Verification items for this drawing (mm, ordinates from the low corner). A direction names the side the tool comes from. Coordinates: 2 decimals unless noted, no trailing zeros. Order: outer loops, then holes, each group sorted by start corner. A loop starts at its lowest first (then second) coordinate and runs counter-clockwise, first axis right, second up. Notation, with made-up numbers: M -22.75,30.25 L 4.25,30.25 A21 cw 4.25,35.25 Z; hole C -32,-3.75 d5. An arc over 180 degrees is marked long. Write item = value, one per line.
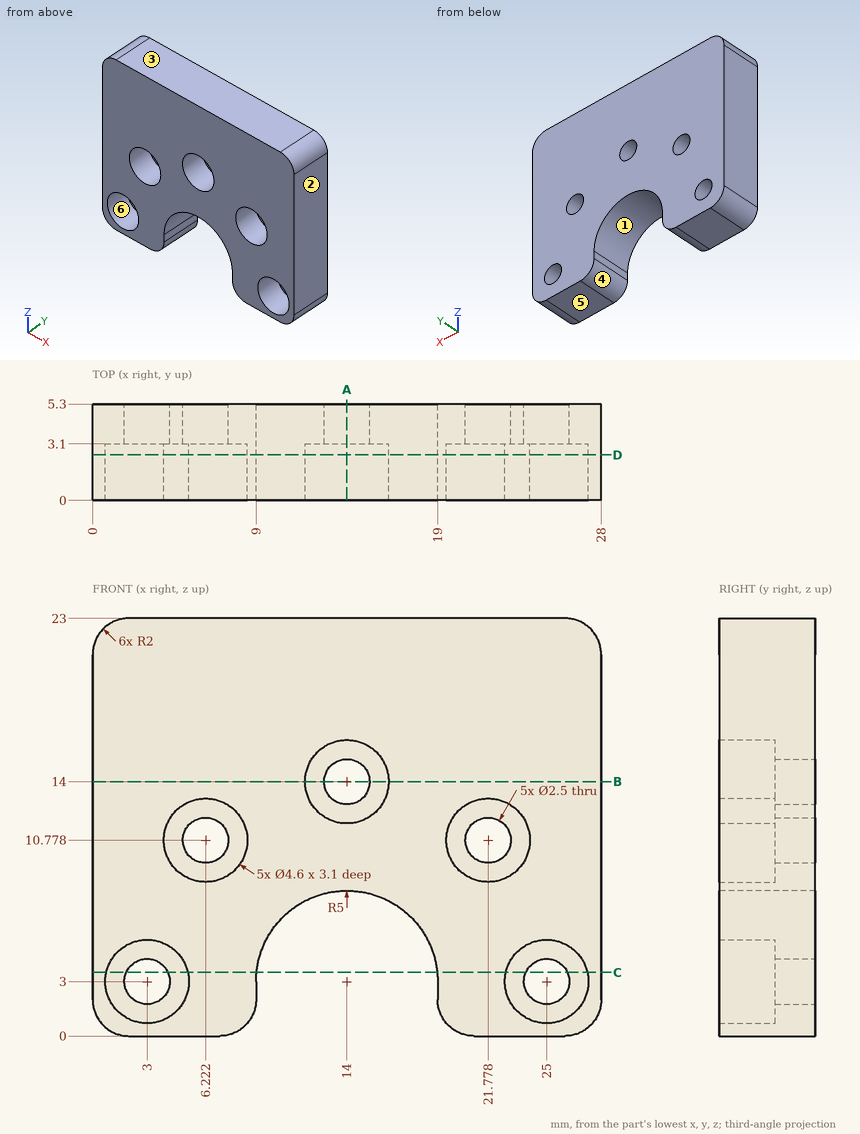
Item 1: Tool access check on the marked faces 4, 5 and 6. Record the directions out of +Z, -Z, +X, -X, +Y, -Y that give a thin tool (end or side, any length) a straight path to the whole face; none if there is none.
Report:
face_4 = -Z, +Y, -Y
face_5 = -Z, +X, -X, +Y, -Y
face_6 = -Y
Item 2: Release check for a two-part mould opening along X. For the marked faces 1, 2 and 3 record: pulls with the +X half, pulls with the -X half, needs draft (parallel to the pull), parting line crosses it, or undercut.
Report:
face_1 = undercut
face_2 = pulls with the +X half
face_3 = needs draft
Item 3: Sectioned sample at A-A, the plane x = 14. Enter the section's corners in (y, z).
Report:
outline = M 0,8 L 5.3,8 L 5.3,12.75 L 3.1,12.75 L 3.1,11.7 L 0,11.7 Z; M 0,16.3 L 3.1,16.3 L 3.1,15.25 L 5.3,15.25 L 5.3,23 L 0,23 Z
Item 4: Sectioned sample at C-C, the plane z = 3.5. Enter the section's corners in (x, y) (1 decimal).
Report:
outline = M 0,0 L 0.8,0 L 0.8,3.1 L 1.9,3.1 L 1.9,5.3 L 0,5.3 Z; M 4.1,3.1 L 5.2,3.1 L 5.2,0 L 9,0 L 9,5.3 L 4.1,5.3 Z; M 19,0 L 22.8,0 L 22.8,3.1 L 23.9,3.1 L 23.9,5.3 L 19,5.3 Z; M 26.1,3.1 L 27.2,3.1 L 27.2,0 L 28,0 L 28,5.3 L 26.1,5.3 Z
Item 5: Sectioned sample at B-B, the plane z = 14. Enter the section's corners in (x, y).
Report:
outline = M 0,0 L 11.7,0 L 11.7,3.1 L 12.75,3.1 L 12.75,5.3 L 0,5.3 Z; M 15.25,3.1 L 16.3,3.1 L 16.3,0 L 28,0 L 28,5.3 L 15.25,5.3 Z
Item 6: Sectioned sample at D-D, the plane y = 2.5. Enter the section's corners in (x, z).
Report:
outline = M 0,2 A2 ccw 2,0 L 7,0 A2 ccw 9,2 L 9,3 A5 cw 19,3 L 19,2 A2 ccw 21,0 L 26,0 A2 ccw 28,2 L 28,21 A2 ccw 26,23 L 2,23 A2 ccw 0,21 Z; hole C 3,3 d4.6; hole C 6.22,10.78 d4.6; hole C 14,14 d4.6; hole C 21.78,10.78 d4.6; hole C 25,3 d4.6
Item 7: Scan lines: L1, parallel to Z at x = 14, y = 4.3; L2, parallel to X at y = 0.95, z = 3; L3, parallel to Z at x = 3, y = 1.25. Record each from-to range of solid material in increasing order. Write a range as from..to.
Report:
L1 = 8..12.75, 15.25..23
L2 = 0..0.7, 5.3..9, 19..22.7, 27.3..28
L3 = 0..0.7, 5.3..23
Item 8: Gauge pin test, flat ends, axial feed: pin 1 (2.5 mm diameter, centred on x = 14.5, z = 14, fed in from -Y); pin 2 (2 mm diameter, centred on x = 9.5, y = 3.5, fed in from -Z); pin 3 (2 mm diameter, centred on x = 8.5, y = 2.5, fed in from -Z). Record the tip position at first contact, or that the pin passes through.
Report:
pin_1 = 3.1
pin_2 = 0.68
pin_3 = 0.06
